```python
from build123d import *

# Parameters (mm, degrees)
BOSS_EXTRUDE1_DEPTH = 3


with BuildPart() as part:
    # Sketch1 → Boss-Extrude1 (new body)
    with BuildSketch(Plane.XY.offset(10)):
        Polygon((12.5, -13), (12.5, -10), (22.5, -10), (22.5, -13), (32.5, -13), (32.5, -10), (42.5, -10), (42.5, -13), (52.5, -13), (52.5, -10), (62.5, -10), (62.5, -13), (72.5, -13), (72.5, -10), (82.5, -10), (82.5, -13), (92.5, -13), (92.5, -10), (102.5, -10), (102.5, -13), (112.5, -13), (112.5, -10), (122.5, -10), (122.5, -13), (132.5, -13), (132.5, -10), (142.5, -10), (142.5, -13), (152.5, -13), (152.5, -10), (165, -10), (165, 0), (168, 0), (168, 10), (165, 10), (165, 20), (168, 20), (168, 30), (165, 30), (165, 40), (168, 40), (168, 50), (165, 50), (165, 60), (168, 60), (168, 70), (165, 70), (165, 80), (168, 80), (168, 90), (165, 90), (165, 100), (168, 100), (168, 110), (165, 110), (165, 120), (168, 120), (168, 130), (165, 130), (165, 140), (152.5, 140), (152.5, 143), (142.5, 143), (142.5, 140), (132.5, 140), (132.5, 143), (122.5, 143), (122.5, 140), (112.5, 140), (112.5, 143), (102.5, 143), (102.5, 140), (92.5, 140), (92.5, 143), (82.5, 143), (82.5, 140), (72.5, 140), (72.5, 143), (62.5, 143), (62.5, 140), (52.5, 140), (52.5, 143), (42.5, 143), (42.5, 140), (32.5, 140), (32.5, 143), (22.5, 143), (22.5, 140), (12.5, 140), (12.5, 143), (2.5, 143), (2.5, 140), (-10, 140), (-10, 130), (-13, 130), (-13, 120), (-10, 120), (-10, 110), (-13, 110), (-13, 100), (-10, 100), (-10, 90), (-13, 90), (-13, 80), (-10, 80), (-10, 70), (-13, 70), (-13, 60), (-10, 60), (-10, 50), (-13, 50), (-13, 40), (-10, 40), (-10, 30), (-13, 30), (-13, 20), (-10, 20), (-10, 10), (-13, 10), (-13, 0), (-10, 0), (-10, -10), (2.5, -10), (2.5, -13), align=None)
    extrude(amount=BOSS_EXTRUDE1_DEPTH)


solid = part.part
```
Source: CAD feature listing. Evaluate the final solid. Frame: model axes, mm. Round coordinates to 2 decimals unless told otherwise and drop trailing zeros. Loops run counter-clockwise (first coordinate to the right, second up) from the corner with the lowest first, then second, coordinate; pieces in that order, holes last. Notation, with made-up numbers: M 5,65 L 26,65 A11 cw 26,76 Z; hole C -13.75,48.5 d3. An arc over 180 degrees is marked long. Use a Markdown table: item, result. Add a question column.
1. Cut plane B-B, the plane x = 38.5. Output: boundary loops of the cut face in (y, z).
2. Ray query, line 1 along X through (y, z) = (35.5, 12.6); line 2 along Y through (x, z) = (15, 12.3). Return the intervals inside material, ascending. Write a range as [from, to].
3. Cut plane A-A, the plane y = 14.5. Output: boundary loops of the cut face in (x, z), and give its area (3 significant figures).
4. Contact query for flat-ended pins moving along their axis: pin 1 (1.5 mm diameter, centred on x = 166, z = 12, fed in from -Y); pin 2 (0.9 mm diameter, centred on y = 114.5, z = 11, fed in from +X); pin 3 (1.5 mm diameter, centred on x = -5.5, z = 11.5, fed in from +Y). Output: stop coordinate, or through.
Solution:
| question | item | result |
|---|---|---|
| 1 | outline | M -10,10 L 140,10 L 140,13 L -10,13 Z |
| 2 | line 1 | x = [-10, 165] |
| 2 | line 2 | y = [-10, 140] |
| 3 | outline | M -10,10 L 165,10 L 165,13 L -10,13 Z |
| 3 | area | 525 mm2 |
| 4 | pin 1 | stops at y = 0 |
| 4 | pin 2 | stops at x = 165 |
| 4 | pin 3 | stops at y = 140 |
